```python
from build123d import *

# Parameters (mm, degrees)
SZKIC1_W                   = 6
SZKIC1_H                   = 40
SZKIC2_W                   = 18
SZKIC2_H                   = 8
WYTNIJ_WYCI_GNI_CIE1_DEPTH = 20


with BuildPart() as part:
    # Szkic1 → Obrót1 (revolve)
    with BuildSketch(Plane(origin=(0, 0, 0), x_dir=(1, 0, 0), z_dir=(0, 1, 0))):
        with Locations((3, 20)):
            Rectangle(SZKIC1_W, SZKIC1_H)
        Polygon((0, 0), (0, -25), (9, -25), (9, 0), (6, 0), align=None)
    revolve(axis=Axis((0, 0, 44.409951059), (0, 0, -1)))

    # Szkic2 → Wytnij-wyciągnięcie1 (cut)
    with BuildSketch(Plane.XY.offset(25)):
        Rectangle(SZKIC2_W, SZKIC2_H)
    extrude(amount=-WYTNIJ_WYCI_GNI_CIE1_DEPTH, mode=Mode.SUBTRACT)


solid = part.part
```
Geometry: final body of the model. Coordinates: model frame, mm. A direction names the side the tool comes from. Round coordinates to 2 decimals unless told otherwise and drop trailing zeros. Loops run counter-clockwise (first coordinate to the right, second up) from the corner with the lowest first, then second, coordinate; pieces in that order, holes last. Notation, with made-up numbers: (54.25, 35) -> (88.25, 35) arc R20 ccw to (88.25, 73) -> close; hole circle Ø9 at (53, 34.5). An arc over 180 degrees is marked (long way). Use one line per item in the form item = value. Start each with the question number.
1) Line query: L1, parallel to Y at x = -0.5, z = 17.5; L2, parallel to Z at x = 1, y = 0.5; L3, parallel to Z at x = 6.25, y = -3.5. Output: solid intervals per line, ascending.
2) Section D-D on z = -8.5. Output: boundary loops of the cut face in (x, y).
3) Section B-B on z = 7.5. Output: boundary loops of the cut face in (x, y), then the cut area to 3 significant figures.
4) Section C-C on y = 0. Output: boundary loops of the cut face in (x, z).
5) First-contact query: P1, Ø1.5, axis at x = 4, z = 0, coming from the -Y side; P2, Ø5, axis at y = -1, z = -23.5, coming from the +X side; P3, Ø2, axis at x = 6, z = 0, coming from the +Y side. Flat tips, straight axial feed; report the tip coordinate or a pass-through.
6) Access query for faces 1 (the flat face through (2, 6, 0)), 2 (the flat face through (0, 4, 15)), 3 (the cylindrical face through (-6.633, -6.083, 12.325)). Directions: +Z, -Z, +X, -X, +Y, -Y. A direction counts if a zero-diameter tool reaches every point of the face in a straight line with its end or side. Return the directions, or none.
7) Section A-A on x = 0. Output: boundary loops of the cut face in (y, z), then the cut area to 3 significant figures.
Response:
q1.L1 = -8.99 to -4, 4 to 8.99
q1.L2 = -40 to 5
q1.L3 = 0 to 5
q2.outline = circle Ø12 at (0, 0)
q3.outline = (-8.06, -4) arc R9 ccw to (8.06, -4) -> close; (-8.06, 4) -> (8.06, 4) arc R9 ccw to start
q3.area = 115 mm^2
q4.outline = (-9, 0) -> (-6, 0) -> (-6, -40) -> (6, -40) -> (6, 0) -> (9, 0) -> (9, 5) -> (-9, 5) -> close
q5.P1 = -8.39
q5.P2 = 6
q5.P3 = 7.48
q6.face_1 = -Z
q6.face_2 = +Z, +X, -X
q6.face_3 = +Z, -Z
q7.outline = (-9, 0) -> (-6, 0) -> (-6, -40) -> (6, -40) -> (6, 0) -> (9, 0) -> (9, 25) -> (4, 25) -> (4, 5) -> (-4, 5) -> (-4, 25) -> (-9, 25) -> close
q7.area = 770 mm^2
